Here's the drawing with two shaded views (mm, measured from the low corner). I have some questions. A direction names the side the tool comes from. Give positions to 0.01 mm unless a question says otherwise; leave off trailing zeros. Loops run counter-clockwise (first coordinate to the right, second up) from the corner with the lowest first, then second, coordinate; pieces in that order, holes last. Notation, with made-up numbers: M 25.25,41 L 81.25,41 A26 ccw 81.25,67 Z; hole C 64.5,27.25 d11. An arc over 180 degrees is marked long. Use a Markdown table: item, result. Add a question column.
1) Suppose I cut it at B-B on x = 4. List the corners of the cut face in (y, z) for me.
2) Suppose I cut it at D-D on y = 27.5. List the corners of the cut face in (x, z) for me.
3) If I drill on line 1 along Y through (x, z) = (6.75, 12.5); line 2 along X through (y, z) = (34.9, 44); line 3 along X through (y, z) = (24, 15.5), over which ranges is the centre line in solid material (lowest first)? Write a range as [from, to].
4) Which directions (+Z, -Z, +X, -X, +Y, -Y) give clear straight access to the entire face, cutting with the end or side of a thin tool? Please do the marked faces 1 and 2.
5) Suppose I cut it at A-A on z = 6. List the corners of the cut face in (x, y) for me.
6) Suppose I cut it at C-C on z = 44. List the corners of the cut face in (x, y) for me.
7) Will these pins go through, and if not, where does the flat tip stop? pin 1 Ø2.5 at (x, y) = (2.5, 24.5) entering from -Z; pin 2 Ø2 at (x, y) = (3.5, 22) entering from +Z; pin 3 Ø4 at (x, z) = (5, 40) entering from -Y; pin 4 Ø2 at (x, z) = (4, 44) entering from -Y.
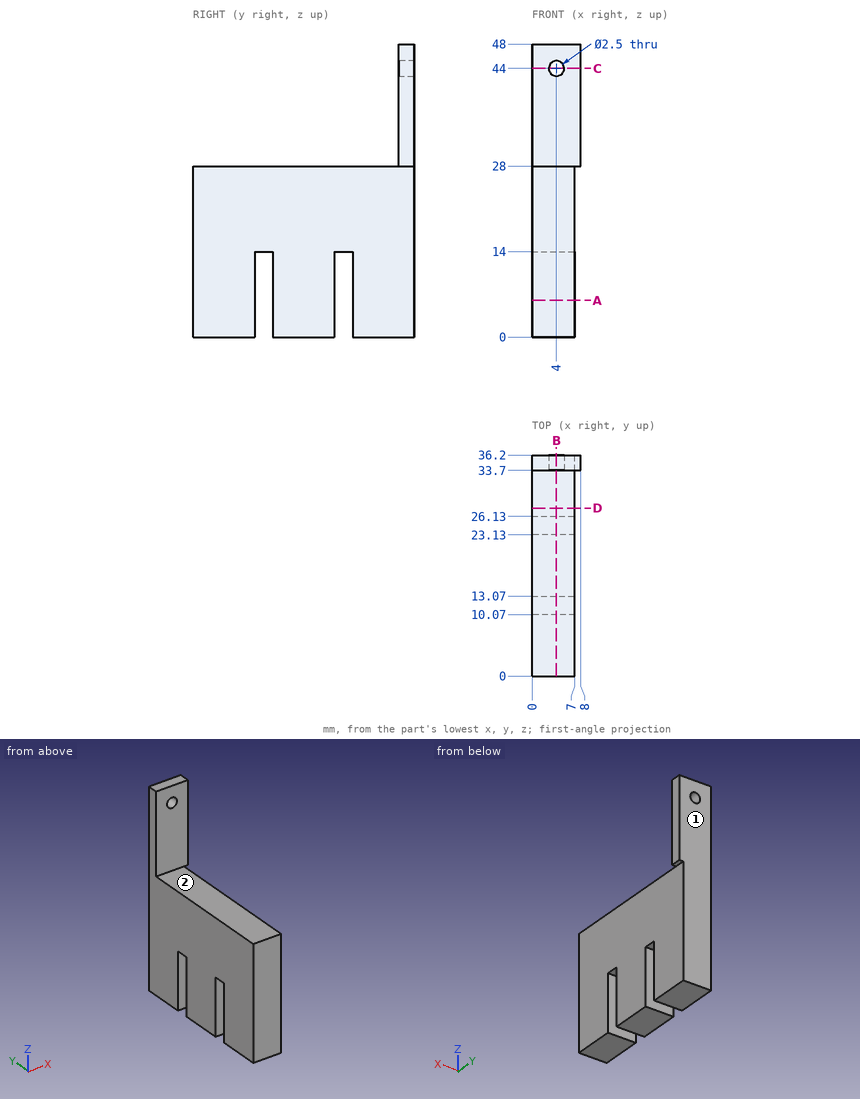
Answer block:
| question | item | result |
|---|---|---|
| 1 | outline | M 0,0 L 10.07,0 L 10.07,14 L 13.07,14 L 13.07,0 L 23.13,0 L 23.13,14 L 26.13,14 L 26.13,0 L 36.2,0 L 36.2,42.75 L 33.7,42.75 L 33.7,28 L 0,28 Z; M 33.7,45.25 L 36.2,45.25 L 36.2,48 L 33.7,48 Z |
| 2 | outline | M 0,0 L 7,0 L 7,28 L 0,28 Z |
| 3 | line 1 | y = [0, 10.07], [13.07, 23.13], [26.13, 36.2] |
| 3 | line 2 | x = [0, 2.75], [5.25, 8] |
| 3 | line 3 | x = [0, 7] |
| 4 | face 1 | +Z, -Z, +X, -X, +Y |
| 4 | face 2 | +Z, +X, -X, -Y |
| 5 | outline | M 0,0 L 7,0 L 7,10.07 L 0,10.07 Z; M 0,13.07 L 7,13.07 L 7,23.13 L 0,23.13 Z; M 0,26.13 L 7,26.13 L 7,36.2 L 0,36.2 Z |
| 6 | outline | M 0,33.7 L 2.75,33.7 L 2.75,36.2 L 0,36.2 Z; M 5.25,33.7 L 8,33.7 L 8,36.2 L 5.25,36.2 Z |
| 7 | pin 1 | stops at z = 14 |
| 7 | pin 2 | stops at z = 28 |
| 7 | pin 3 | stops at y = 33.7 |
| 7 | pin 4 | passes through |
